Input: dimensioned drawing with shaded views. Units: mm. Origin: part minimum x, y, z. Give positions to 0.01 mm unless a question says otherwise; leave off trailing zeros. Order: outer loops, then holes, each group sorted by start corner. A loop starts at its lowest first (then second) coordinate and runs counter-clockwise, first axis right, second up.
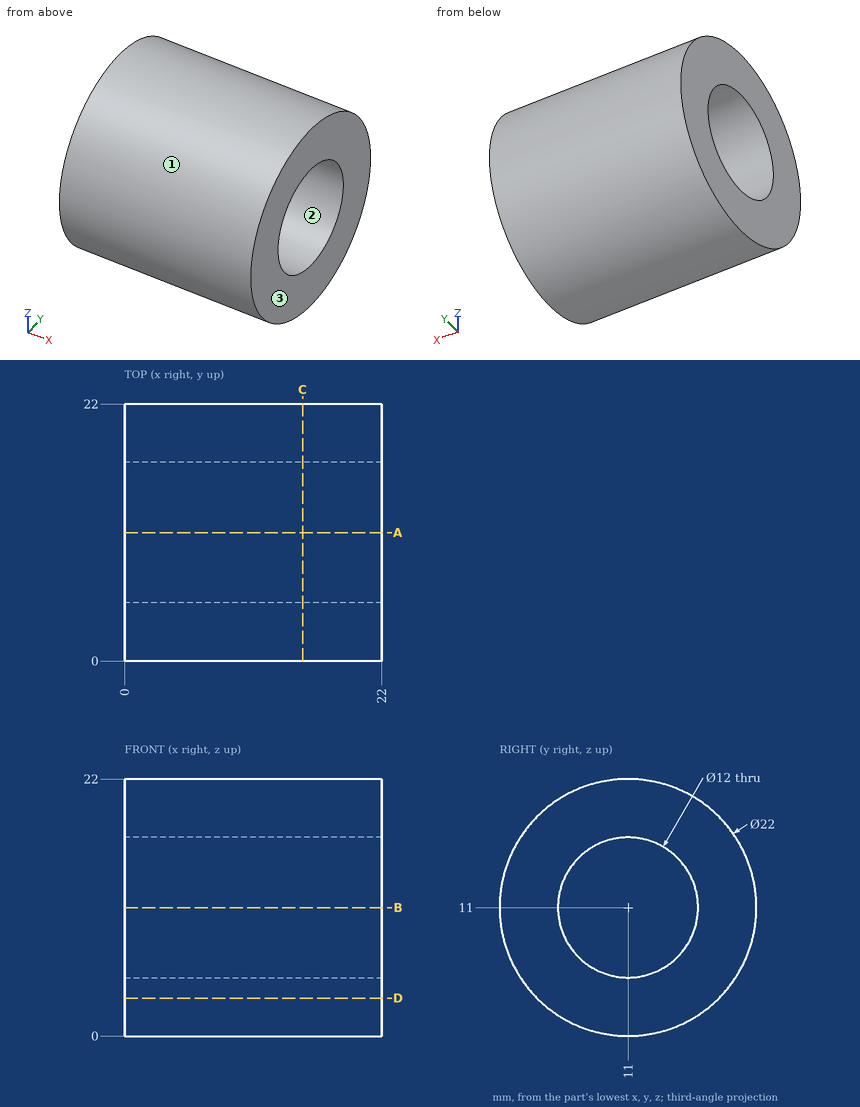
1) Section query D-D, the plane z = 3.25. Return the cut outline in (x, y).
Report:
outline: (0, 3.19) - (22, 3.19) - (22, 18.81) - (0, 18.81) - close
2) Material intervals for L1, parallel to Y at x = 12, z = 11; L2, parallel to Z at x = 17, y = 12; L3, parallel to Z at x = 1, y = 7.5, sorted ascending.
Report:
L1: y = 0 to 5, 17 to 22
L2: z = 0.05 to 5.08, 16.92 to 21.95
L3: z = 0.57 to 6.13, 15.87 to 21.43
3) Section query A-A, the plane y = 11. Return the cut outline in (x, z).
Report:
outline: (0, 0) - (22, 0) - (22, 5) - (0, 5) - close; (0, 17) - (22, 17) - (22, 22) - (0, 22) - close
4) Section query C-C, the plane x = 15.25. Return the cut outline in (y, z).
Report:
outline: circle Ø22 at (11, 11); hole circle Ø12 at (11, 11)
5) Draft query along Z for the marked faces 1, 2 and 3. Return one class per face: +Z half, -Z half, draft (parallel to the pull), parting line (faces both ways), or undercut.
Report:
face 1: parting line
face 2: undercut
face 3: draft
6) Pin query (flat end, axial travel): pin 1 (1.5 mm diameter, centred on x = 6, z = 6, fed in from -Y); pin 2 (3 mm diameter, centred on x = 12.5, y = 16, fed in from -Z); pin 3 (2 mm diameter, centred on x = 18.5, y = 5.5, fed in from -Z). Return the tip coordinate at first contact, or that it passes through.
Report:
pin 1: stops at y = 0.85
pin 2: stops at z = 0.57
pin 3: stops at z = 0.96
